Read the model definition and answer for the solid it produces. Units are mm, in the model's axes. Face numbers are marked on the shaded views. A direction names the side the tool comes from. Coordinates: 2 decimals unless noted, no trailing zeros. Loops run counter-clockwise (first coordinate to the right, second up) from the corner with the lowest first, then second, coordinate; pieces in that order, holes last. Notation, with made-up numbers: (-7, 17.25) -> (15, 17.25) arc R10 cw to (15, 25.25) -> close; hole circle Ø4 at (8, -12.5). An arc over 180 degrees is marked (long way). Answer as a JSON object with one key per item and string values. Group by question number.
1) Consider probe 1 along Z at (x, y) = (-33, 40); probe 2 along Z at (x, y) = (-39, 40); probe 3 along X at (y, z) = (22, 3.25). Determine where each line is inside the solid, lowest interval first. Write a range as [from, to].
2) Section A-A, the plane z = 10 is taken. Give the vertices of the cut face in (x, y).
3) Which of the six approach directions +Z, -Z, +X, -X, +Y, -Y give full straight-line access (tool end or side, diameter ignored) to the marked faces 4 and 5?
4) Determine the mould class of the marked faces 1, 2 and 3 for opening direction X: released by +X, released by -X, zero draft, split by the parting line, or undercut.
5) Section D-D, the plane y = 29 is taken. Give the vertices of the cut face in (x, z), plus the area to 3 significant figures.
6) Flat-ended cylindrical pins translate along their axes: P1, Ø2, axis at x = 1, z = 8, coming from the +Y side; P2, Ø1, axis at x = -5.5, z = 13, coming from the +Y side; P3, Ø4, axis at y = 37.5, z = 15, coming from the +X side; P4, Ø3, axis at y = 40, z = 10, coming from the -X side. Find the tip coordinate at first contact, or state that the pin passes through.
7) Section B-B, the plane y = 40 is taken. Give the vertices of the cut face in (x, z).
8) Section C-C, the plane y = -18.5 is taken. Give the vertices of the cut face in (x, z).
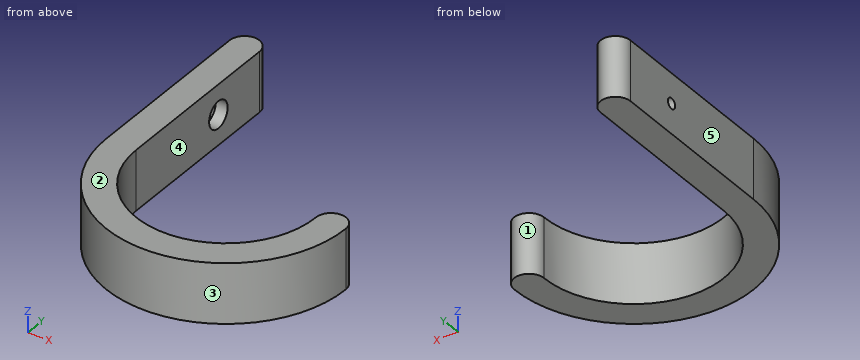
from build123d import *

# Parameters (mm, degrees)
F6_DEPTH = 20
F8_D     = 3.5
F8_DEPTH = 10
F8_TIP   = 1.0515060833
F9_D     = 9
F9_DEPTH = 4
F9_TIP   = 2.7038727856


with BuildPart() as f6:
    # F5 (on Top) → F6 (new body)
    with BuildSketch(Plane.XY):
        with BuildLine():
            ThreePointArc((30, 0), (0, -30), (-30, 0))
            Line((-30, 0), (-30, 60))
            ThreePointArc((-30, 60), (-35, 65), (-40, 60))
            Line((-40, 60), (-40, 0))
            ThreePointArc((-40, 0), (0, -40), (40, 0))
            ThreePointArc((40, 0), (35, 5.0700953218), (30, 0))
        make_face()
    extrude(amount=F6_DEPTH)

    # F8
    with Locations(Plane.YZ.offset(-30)):
        with Locations((40, 10)):
            Hole(F8_D / 2, depth=F8_DEPTH)
            with Locations((0, 0, -(F8_DEPTH + F8_TIP / 2))):  # 118° drill point
                Cone(0, F8_D / 2, F8_TIP, mode=Mode.SUBTRACT)

    # F9
    with Locations(Plane.YZ.offset(-30)):
        with Locations((40, 10)):
            Hole(F9_D / 2, depth=F9_DEPTH)
            with Locations((0, 0, -(F9_DEPTH + F9_TIP / 2))):  # 118° drill point
                Cone(0, F9_D / 2, F9_TIP, mode=Mode.SUBTRACT)


solid = f6.part
Determined:
{
 "1": {"probe 1": "[0, 5.5], [14.5, 20]", "probe 2": "[0, 8.25], [11.75, 20]", "probe 3": "[-40, -30]"},
 "2": {"outline": "(-40, 0) arc R40 ccw to (40, 0) arc R5 ccw (long way) to (30, 0) arc R30 cw to (-30, 0) -> (-30, 35.5) -> (-34, 35.5) -> (-35.65, 38.25) -> (-40, 38.25) -> close; (-40, 41.75) -> (-35.65, 41.75) -> (-34, 44.5) -> (-30, 44.5) -> (-30, 60) arc R5 ccw to (-40, 60) -> close"},
 "3": {"face 4": "+Z, -Z, +Y", "face 5": "+Z, -Z, -X, +Y, -Y"},
 "4": {"face 1": "undercut", "face 2": "zero draft", "face 3": "split by the parting line"},
 "5": {"outline": "(-40, 0) -> (-30, 0) -> (-30, 20) -> (-40, 20) -> close", "area": "200 mm²"},
 "6": {"P1": "y = -29.93", "P2": "y = -29.39", "P3": "x = -30", "P4": "through"},
 "7": {"outline": "(-40, 0) -> (-30, 0) -> (-30, 5.5) -> (-34, 5.5) -> (-35.65, 8.25) -> (-40, 8.25) -> close; (-40, 11.75) -> (-35.65, 11.75) -> (-34, 14.5) -> (-30, 14.5) -> (-30, 20) -> (-40, 20) -> close"},
 "8": {"outline": "(-35.46, 0) -> (-23.62, 0) -> (-23.62, 20) -> (-35.46, 20) -> close; (23.62, 0) -> (35.46, 0) -> (35.46, 20) -> (23.62, 20) -> close"}
}
